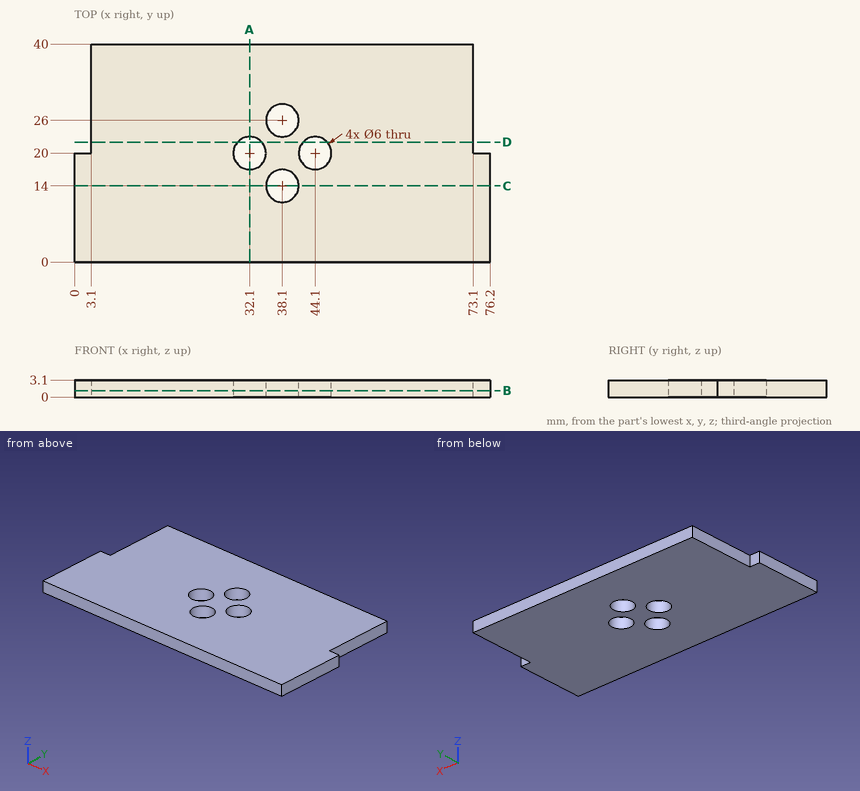
Geometry: see drawing. Coordinates: mm, zero at the bounding-box minimum. Coordinates: 2 decimals unless noted, no trailing zeros. Order: outer loops, then holes, each group sorted by start corner. A loop starts at its lowest first (then second) coordinate and runs counter-clockwise, first axis right, second up. Notation, with made-up numbers: M -29.5,78 L 16.5,78 A22 ccw 16.5,114 Z; hole C -20,30.25 d1. An arc over 180 degrees is marked long. Answer in a Markdown table with one row per item. Add a question column.
Q1. Section query C-C on y = 14. Return the cut outline in (x, z).
Q2. Contact query for flat-ended pins moving along their axis: P1, Ø0.9, axis at x = 74, z = 1.5, coming from the +Y side; P2, Ø5.5, axis at x = 38.1, y = 14, coming from the -Z side; P3, Ø1.5, axis at y = 34, z = 1.5, coming from the -X side. Output: stop coordinate, or through.
Q3. Line query: L1, parallel to Y at x = 38.1, z = 2.1; L2, parallel to Y at x = 44.1, z = 2.25; L3, parallel to X at y = 30, z = 1.55. Output: solid intervals per line, ascending.
Q4. Section query B-B on z = 1.2. Return the cut outline in (x, y), and give its area (3 significant figures).
Q5. Section query A-A on x = 32.1. Return the cut outline in (y, z).
Q6. Section query D-D on y = 22. Return the cut outline in (x, z).
Completed:
| question | item | result |
|---|---|---|
| 1 | outline | M 0,0 L 35.1,0 L 35.1,3.1 L 0,3.1 Z; M 41.1,0 L 76.2,0 L 76.2,3.1 L 41.1,3.1 Z |
| 2 | P1 | stops at y = 20 |
| 2 | P2 | passes through |
| 2 | P3 | stops at x = 3.1 |
| 3 | L1 | y = 0 to 11, 17 to 23, 29 to 40 |
| 3 | L2 | y = 0 to 17, 23 to 40 |
| 3 | L3 | x = 3.1 to 73.1 |
| 4 | outline | M 0,0 L 76.2,0 L 76.2,20 L 73.1,20 L 73.1,40 L 3.1,40 L 3.1,20 L 0,20 Z; hole C 32.1,20 d6; hole C 38.1,14 d6; hole C 38.1,26 d6; hole C 44.1,20 d6 |
| 4 | area | 2,810 mm2 |
| 5 | outline | M 0,0 L 17,0 L 17,3.1 L 0,3.1 Z; M 23,0 L 40,0 L 40,3.1 L 23,3.1 Z |
| 6 | outline | M 3.1,0 L 29.86,0 L 29.86,3.1 L 3.1,3.1 Z; M 34.34,0 L 41.86,0 L 41.86,3.1 L 34.34,3.1 Z; M 46.34,0 L 73.1,0 L 73.1,3.1 L 46.34,3.1 Z |
